Here's how the part is built. I have some questions about the finished solid (model axes, mm). A direction names the side the tool comes from. Coordinates: 2 decimals unless noted, no trailing zeros. Write each loop counter-clockwise with the first axis right and the second up, starting at its lowest first coordinate (ties: lowest second). Pieces come first, ordered by that corner, then holes. Notation, with made-up numbers: (86.5, 44) - (141.5, 44) arc R31 ccw to (141.5, 76) - close; hole circle Ø5 at (39.5, 6). An arc over 180 degrees is marked (long way). Answer in a Markdown table with one row per item. Add a question column.
Item 1: I'm going to push flat-ended pins straight in: pin 1 (10 mm diameter, centred on x = -1, z = -15, fed in from +Y); pin 2 (8.5 mm diameter, centred on y = 12, z = -10.5, fed in from +X); pin 3 (1.3 mm diameter, centred on x = 22.5, z = 29.5, fed in from +Y). Where does each tip first touch, or does it pass through?
Item 2: We'd pull the mould along Y, two halves only. Please class faces 1 (the face through (23, 16, 33.213)), 2 (the face through (27, 30.5, -41)), 3 (the face through (52.07, 24.97, 31.98)): +Y half, -Y half, draft (parallel to the pull), parting line (faces both ways), or undercut.
Item 3: Which directions (+Z, -Z, +X, -X, +Y, -Y) give clear straight access to the entire face, cutting with the end or side of a thin tool? Please do faces 4 (the face through (62.301, 24.967, 21.713)), 5 (the face through (62.34, 6.3, 7.59)), 6 (the face through (25, 23.5, -42)), 7 (the face through (15, 12.5, -39)).
Item 4: If I drill on probe 1 along Y at (x, z) = (2, 32.5); probe 2 along Z at (x, y) = (62.7, 27.25); probe 3 along X at (y, z) = (7.5, 7.5), over which ranges is the centre line in solid material (lowest first)? Write a range as from..to.
Item 5: Imagine slicing it at A-A (y = 25). Please give me the cut outline in (x, z).
Item 6: Imagine slicing it at B-B (z = -24.5). State how many separate pieces and enclosed holes the cut face has, plus the area to 3 significant figures.
Item 7: Imagine slicing it at D-D (y = 8.5). Please give me the cut outline in (x, z), plus the area to 3 significant figures.
Autodesk Inventor part; units mm, degrees
ref_plane "YZ Plane" through (0, 0, 0) normal (1, 0, 0) x (0, 1, 0)
ref_plane "XZ Plane" through (0, 0, 0) normal (0, 1, 0) x (-1, 0, 0)
ref_plane "XY Plane" through (0, 0, 0) normal (0, 0, 1) x (1, 0, 0)
sketch "Skizze1" plane through (0, 0, 0) normal (0, 1, 0) x (-1, 0, 0)
  line L0 (16.4314, 33.2132) -> (-63.5686, 33.2132)
  line L1 (-63.5686, 33.2132) -> (-63.5686, -42.7868)
  line L2 (-63.5686, -42.7868) -> (16.4314, -42.7868)
  line L3 (16.4314, -42.7868) -> (16.4314, 33.2132)
  point P0 (0, 0)
  dimension "d0" = 76
  dimension "d1" = 80
extrude "Extrusion1" add sketch "Skizze1" along normal blind 30.5
shell "Wandung1" thickness 2.5 removed faces 1 at (36.9019, 30.5, 7.8799)
sketch "Skizze2" plane through (-13.9314, 2.5, -40.2868) normal (0, 1, 0) x (1, 0, 0)
  line L0 (0, -71) -> (0, 0)
  line L1 (75, 0) -> (75, -71)
  line L2 (75, -71) -> (75, 0)
  line L3 (0, 0) -> (0, -71)
  line L4 (0, -71) -> (0, -66.5)
  line L5 (0, -66.5) -> (20, -66.5)
  line L6 (20, -66.5) -> (20, -69)
  line L7 (20, -69) -> (75, -69)
  line L8 (75, -69) -> (75, -71)
  line L9 (0, -71) -> (75, -71)
  line L10 (0, -35.5) -> (75, -35.5)
  line L11 (0, 0) -> (0, -4.5)
  line L12 (0, -4.5) -> (20, -4.5)
  line L13 (20, -4.5) -> (20, -2)
  line L14 (20, -2) -> (75, -2)
  line L15 (75, -2) -> (75, 0)
  line L16 (0, 0) -> (75, 0)
  point P0 (75, 0)
  point P1 (75, -2)
  point P2 (0, -4.5)
  point P3 (0, -66.5)
  dimension "d35" = 4.5
  dimension "d36" = 2
  dimension "d37" = 20
extrude "Extrusion2" add sketch "Skizze2" along normal blind 10 contours L0 L5 L6 L7 L1 L9 | L0 L16 L1 L14 L13 L12
sketch "Skizze3" plane through (-13.9314, 12.5, -40.2868) normal (0, 1, 0) x (1, 0, 0)
  circle A0 centre (2.25, -68.75) radius 0.75
  line L0 (2.25, -68.75) -> (2.25, -66.5) construction
  line L1 (2.25, -68.75) -> (0, -68.75) construction
  line L2 (0, -71) -> (0, 0) construction
  line L3 (75, 0) -> (75, -71) construction
  line L4 (75, -71) -> (0, -71) construction
  circle A1 centre (2.25, -2.25) radius 0.75
  line L5 (0, 0) -> (75, 0)
  point P0 (13.9314, -40.2868)
  dimension "d8" = 1.5
  dimension "d14" = 2.25
  dimension "d38" = 2.25
  dimension "d39" = 2.25
  dimension "d40" = 2.25
extrude "Extrusion3" cut sketch "Skizze3" against normal blind 8
sketch "Skizze6" plane through (63.5686, 0, 33.2132) normal (1, 0, 0) x (0, 0, -1)
  line L0 (69.5, 10) -> (69.5, 2.75)
  line L1 (0, 0) -> (76, 0)
  line L2 (76, 0) -> (76, 30.5)
  line L3 (0, 0) -> (0, 30.5)
  line L4 (10, 6.375) -> (22, 6.375) construction
  line L5 (10, 2.75) -> (22, 2.75)
  line L6 (22, 10) -> (10, 10)
  arc A0 (10, 10) -> (10, 2.75) centre (10, 6.375) ccw
  arc A1 (22, 2.75) -> (22, 10) centre (22, 6.375) ccw
  line L7 (54, 6.375) -> (66, 6.375) construction
  line L8 (54, 2.75) -> (66, 2.75)
  line L9 (66, 10) -> (54, 10)
  arc A2 (54, 10) -> (54, 2.75) centre (54, 6.375) ccw
  arc A3 (66, 2.75) -> (66, 10) centre (66, 6.375) ccw
  point P0 (33.2132, 0)
  point P1 (16, 6.375)
  point P2 (60, 6.375)
  point P3 (69.5, 5.4313)
  point P4 (69.5, 7.3187)
  dimension "d31" = 6.5
  dimension "d59" = 7.25
  dimension "d60" = 2.75
  dimension "d61" = 10
  dimension "d62" = 12
  dimension "d63" = 7.25
  dimension "d64" = 12
  dimension "d65" = 2.75
  dimension "d66" = 10
extrude "Extrusion6" cut sketch "Skizze6" against normal blind 10 contours L0 A3 L8 A2 L9 | A0 L6 A1 L5
sketch "Skizze8" plane through (-13.9314, 30.5, 30.7132) normal (1, 0, 0) x (0, 0, -1)
  circle A0 centre (3.2, -3.25) radius 0.75
  circle A1 centre (67.8, -3.25) radius 0.75
  line L0 (0, -18) -> (0, 0)
  line L1 (0, 0) -> (71, 0)
  line L2 (71, -18) -> (71, 0)
  line L3 (10.5, -5.5) -> (60.5, -5.5) construction
  line L4 (10.5, -4) -> (60.5, -4)
  line L5 (60.5, -7) -> (10.5, -7)
  arc A2 (10.5, -4) -> (10.5, -7) centre (10.5, -5.5) ccw
  arc A3 (60.5, -7) -> (60.5, -4) centre (60.5, -5.5) ccw
  line L6 (10.5, -11.5) -> (60.5, -11.5) construction
  line L7 (10.5, -10) -> (60.5, -10)
  line L8 (60.5, -13) -> (10.5, -13)
  arc A4 (10.5, -10) -> (10.5, -13) centre (10.5, -11.5) ccw
  arc A5 (60.5, -13) -> (60.5, -10) centre (60.5, -11.5) ccw
  point P0 (30.7132, -30.5)
  point P1 (35.5, -5.5)
  point P2 (35.5, -11.5)
  dimension "d43" = 1.5
  dimension "d44" = 3.2
  dimension "d45" = 3.25
  dimension "d46" = 3.2
  dimension "d47" = 3.25
  dimension "d50" = 3
  dimension "d51" = 4
  dimension "d53" = 50
  dimension "d54" = 3
  dimension "d55" = 50
  dimension "d56" = 35.5
  dimension "d57" = 3
  dimension "d58" = 35.5
extrude "Extrusion7" cut sketch "Skizze8" along normal through all both and the other way through all
sketch "Skizze9" plane through (61.0686, 30.5, 30.7132) normal (0, 0, -1) x (-1, 0, 0)
  line L0 (10.5, -5.5) -> (60.5, -5.5) construction
  line L1 (77.5, 0) -> (-2.5, 0)
  line L2 (10.5, -4) -> (60.5, -4)
  line L3 (60.5, -7) -> (10.5, -7)
  arc A0 (10.5, -4) -> (10.5, -7) centre (10.5, -5.5) ccw
  arc A1 (60.5, -7) -> (60.5, -4) centre (60.5, -5.5) ccw
  line L4 (0, -18) -> (0, 0)
  line L5 (10.5, -11.5) -> (60.5, -11.5) construction
  line L6 (10.5, -10) -> (60.5, -10)
  line L7 (60.5, -13) -> (10.5, -13)
  arc A2 (10.5, -10) -> (10.5, -13) centre (10.5, -11.5) ccw
  arc A3 (60.5, -13) -> (60.5, -10) centre (60.5, -11.5) ccw
  point P0 (61.0686, -30.5)
  point P1 (35.5, -5.5)
  point P2 (35.5, -11.5)
  dimension "d67" = 50
  dimension "d68" = 35.5
  dimension "d69" = 3
  dimension "d70" = 4
  dimension "d71" = 50
  dimension "d72" = 3
  dimension "d73" = 35.5
  dimension "d74" = 3
extrude "Extrusion8" cut sketch "Skizze9" along normal through all both and the other way through all
sketch "Skizze10" plane through (-16.4314, 0, 33.2132) normal (0, 0, 1) x (1, 0, 0)
  line L0 (0, 0) -> (0, 30.5)
  line L1 (80, 0) -> (0, 0)
  line L2 (0, 0) -> (0, 6.5)
  line L3 (0, 6.5) -> (80, 6.5)
  line L4 (80, 6.5) -> (80, 0)
  point P0 (16.4314, 0)
  dimension "d77" = 6.5
extrude "Extrusion9" add sketch "Skizze10" along normal blind 4
sketch "Skizze11" plane through (63.5686, 0, -42.7868) normal (0, 0, -1) x (-1, 0, 0)
  line L0 (0, 0) -> (0, 30.5)
  line L1 (80, 0) -> (80, 30.5)
  line L2 (0, 0) -> (80, 0)
  line L3 (80, 0) -> (80, 6.5)
  line L4 (80, 6.5) -> (0, 6.5)
  line L5 (0, 6.5) -> (0, 0)
  point P0 (63.5686, 0)
  point P1 (0, 6.5)
  dimension "d80" = 6.5
extrude "Extrusion10" add sketch "Skizze11" along normal blind 4
sketch "Skizze12" plane through (-16.4314, 30.5, -42.7868) normal (-1, 0, 0) x (0, 0, 1)
  line L0 (80, -30.5) -> (-4, -30.5)
  line L1 (76, -24) -> (80, -24)
  line L2 (-4, -30.5) -> (80, -30.5)
  line L3 (80, -30.5) -> (80, -24)
  line L4 (80, -24) -> (-4, -24)
  line L5 (-4, -24) -> (-4, -30.5)
  point P0 (42.7868, -30.5)
extrude "Extrusion11" add sketch "Skizze12" along normal blind 4
sketch "Skizze13" plane through (63.5686, 30.5, 33.2132) normal (1, 0, 0) x (0, 0, -1)
  line L0 (33.625, -24) -> (42.375, -24)
  line L1 (42.375, -24) -> (42.375, -30.5)
  line L2 (42.375, -30.5) -> (33.625, -30.5)
  line L3 (33.625, -30.5) -> (33.625, -24)
  line L4 (-4, -30.5) -> (80, -30.5)
  arc A0 (22, -27.75) -> (22, -20.5) centre (22, -24.125) ccw
  point P0 (33.2132, -30.5)
  dimension "d85" = 6.5
  dimension "d86" = 8.75
  dimension "d87" = 15.25
extrude "Extrusion12" add sketch "Skizze13" along normal blind 4
chamfer "Fase1" distance 2 angle 60 4 edges at (21.5686, 0, 37.2132) (-20.4314, 0, -4.7868) (21.5686, 0, -46.7868) (67.5686, 0, -4.7868) measured on face at (7.5686, 0, -3.3285)
properties part number "GameFrameRaspiBox1"
Here are the results:
| question | item | result |
|---|---|---|
| 1 | pin 1 | stops at y = 2.5 |
| 1 | pin 2 | stops at x = 63.57 |
| 1 | pin 3 | stops at y = 12.5 |
| 2 | face 1 | draft |
| 2 | face 2 | +Y half |
| 2 | face 3 | undercut |
| 3 | face 4 | +X, -X |
| 3 | face 5 | +X |
| 3 | face 6 | +Z, -Z |
| 3 | face 7 | +Y |
| 4 | probe 1 | y = 0..17.5, 20.5..23.5, 26.5..30.5 |
| 4 | probe 2 | z = -42.79..-37.84, -36.34..26.76, 28.26..33.21 |
| 4 | probe 3 | x = -16.43..-13.93, 61.07..63.57 |
| 5 | outline | (-16.43, -42.79) - (-0.93, -42.79) - (-0.93, -40.29) - (-13.93, -40.29) - (-13.93, -31.29) - (-16.43, -31.29) - close; (-16.43, 21.71) - (-13.93, 21.71) - (-13.93, 30.71) - (-0.93, 30.71) - (-0.93, 33.21) - (-16.43, 33.21) - close; (52.07, -42.79) - (63.57, -42.79) - (63.57, -31.29) - (61.07, -31.29) - (61.07, -40.29) - (52.07, -40.29) - close; (52.07, 30.71) - (61.07, 30.71) - (61.07, 21.71) - (63.57, 21.71) - (63.57, 33.21) - (52.07, 33.21) - close |
| 6 | separate pieces | 6 |
| 6 | enclosed holes | 0 |
| 6 | area | 314 mm2 |
| 7 | outline | (-16.43, -42.79) - (63.57, -42.79) - (63.57, -35.72) - (61.07, -35.72) - (61.07, -38.29) - (6.07, -38.29) - (6.07, -35.79) - (-13.93, -35.79) - (-13.93, 26.21) - (6.07, 26.21) - (6.07, 28.71) - (61.07, 28.71) - (61.07, 26.15) - (63.57, 26.15) - (63.57, 33.21) - (-16.43, 33.21) - close; (61.07, -17.85) - (63.57, -17.85) - (63.57, 8.28) - (61.07, 8.28) - close; hole circle Ø1.5 at (-11.68, -38.04); hole circle Ø1.5 at (-11.68, 28.46) |
| 7 | area | 1,060 mm2 |
